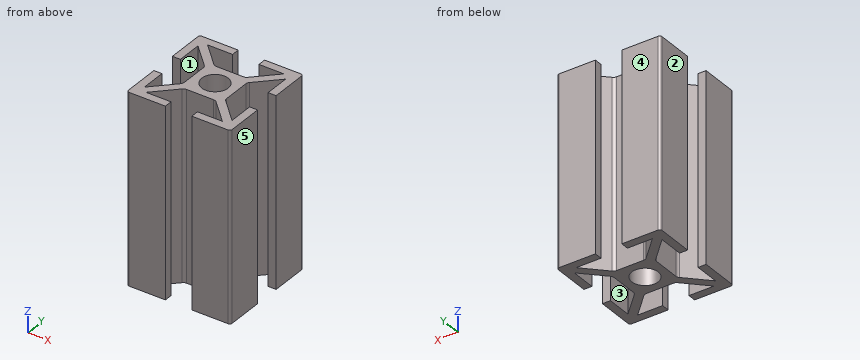
```python
from build123d import *

# Parameters (mm, degrees)
EXTRUSION1_DEPTH        = 40
ESQUISSE2_R             = 2.8
ENL_V_MAT_EXTRU_1_DEPTH = 41
CONG_1_R                = 0.5
CONG_2_R                = 1


with BuildPart() as part:
    # Esquisse1 → Extrusion1 (new body)
    with BuildSketch(Plane.XY):
        Polygon((-2.8, 11), (-2.8, 9.3), (-8.097918472, 9.3), (-3.297918472, 4.5), (3.297918472, 4.5), (8.097918472, 9.3), (2.8, 9.3), (2.8, 11), (11, 11), (11, 2.8), (9.3, 2.8), (9.3, 8.097918472), (4.5, 3.297918472), (4.5, -3.297918472), (9.3, -8.097918472), (9.3, -2.8), (11, -2.8), (11, -11), (2.8, -11), (2.8, -9.3), (8.097918472, -9.3), (3.297918472, -4.5), (-3.297918472, -4.5), (-8.097918472, -9.3), (-2.8, -9.3), (-2.8, -11), (-11, -11), (-11, -2.8), (-9.3, -2.8), (-9.3, -8.097918472), (-4.5, -3.297918472), (-4.5, 3.297918472), (-9.3, 8.097918472), (-9.3, 2.8), (-11, 2.8), (-11, 11), align=None)
    extrude(amount=EXTRUSION1_DEPTH)

    # Esquisse2 → Enlèv. mat.-Extru.1 (cut, through all)
    with BuildSketch(Plane(origin=(0, 0, 0), x_dir=(-1, 0, 0), z_dir=(0, 0, -1))):
        Circle(ESQUISSE2_R)
    extrude(amount=-ENL_V_MAT_EXTRU_1_DEPTH, mode=Mode.SUBTRACT)

    # Congé1
    cong_1_edges = [part.edges().sort_by_distance(p)[0] for p in [
        (-11, 11, 20),
        (11, 11, 20),
        (11, -11, 20),
        (-11, -11, 20),
    ]]
    fillet(cong_1_edges, radius=CONG_1_R)

    # Congé2
    cong_2_edges = [part.edges().sort_by_distance(p)[0] for p in [
        (-4.5, -3.297918472, 20),
        (-4.5, 3.297918472, 20),
        (-3.297918472, 4.5, 20),
        (3.297918472, 4.5, 20),
        (4.5, 3.297918472, 20),
        (4.5, -3.297918472, 20),
        (3.297918472, -4.5, 20),
        (-3.297918472, -4.5, 20),
    ]]
    fillet(cong_2_edges, radius=CONG_2_R)


solid = part.part
```
The model under review builds one solid part; all positions refer to its coordinate system, in mm. Face numbers are marked on the shaded views. A direction names the side the tool comes from. Round coordinates to 2 decimals unless told otherwise and drop trailing zeros. Loops run counter-clockwise (first coordinate to the right, second up) from the corner with the lowest first, then second, coordinate; pieces in that order, holes last. Notation, with made-up numbers: (76, -36.75) -> (110, -36.75) arc R12 ccw to (110, -32.75) -> close; hole circle Ø8 at (-0.75, -32.75). An arc over 180 degrees is marked (long way). Answer as a JSON object with one key per item and string values. Group by question number.
1) We need section C-C on x = -4. Write out the cut boundary in (y, z), then the cut area to 3 significant figures.
2) We need section D-D on y = -6.25. Write out the cut boundary in (x, z).
3) For line 1 (Y direction, x = 0, z = 21); line 2 (Y direction, x = 4.75, z = 22); line 3 (Y direction, x = -3.75, z = 33.5), list the stretches that pass through material, from the lowest coordinate up. Write a range as [from, to].
4) For the marked faces 1 and 2, list the 3-axis set-ups (+Z, -Z, +X, -X, +Y, -Y) from which the entire face can be reached by the end or side of a thin tool; tool diameter is ignored.
5) For pin 1 Ø3 at (x, z) = (1, 27.5) entering from -Y, flat-tipped, find the tip position at first contact; note if it passes through.
6) We need section A-A on y = 0. Write out the cut boundary in (x, z), then the cut area to 3 significant figures.
7) Mouldability with a two-part tool opening along X and no side actions: class the marked faces 3, 4 and 5 as released by +X, released by -X, zero draft, split by the parting line, or undercut.
Result set:
{
 "1": {"outline": "(-11, 0) -> (-9.3, 0) -> (-9.3, 40) -> (-11, 40) -> close; (-5.2, 0) -> (5.2, 0) -> (5.2, 40) -> (-5.2, 40) -> close; (9.3, 0) -> (11, 0) -> (11, 40) -> (9.3, 40) -> close", "area": "552 mm²"},
 "2": {"outline": "(-11, 0) -> (-9.3, 0) -> (-9.3, 40) -> (-11, 40) -> close; (-7.45, 0) -> (-5.05, 0) -> (-5.05, 40) -> (-7.45, 40) -> close; (5.05, 0) -> (7.45, 0) -> (7.45, 40) -> (5.05, 40) -> close; (9.3, 0) -> (11, 0) -> (11, 40) -> (9.3, 40) -> close"},
 "3": {"line 1": "[-4.5, -2.8], [2.8, 4.5]", "line 2": "[-11, -9.3], [-5.95, -3.55], [3.55, 5.95], [9.3, 11]", "line 3": "[-11, -9.3], [-4.95, 4.95], [9.3, 11]"},
 "4": {"face 1": "+Z, -Z", "face 2": "+Z, -Z, -X, +Y, -Y"},
 "5": {"pin 1": "y = -4.5"},
 "6": {"outline": "(-4.5, 0) -> (-2.8, 0) -> (-2.8, 40) -> (-4.5, 40) -> close; (2.8, 0) -> (4.5, 0) -> (4.5, 40) -> (2.8, 40) -> close", "area": "136 mm²"},
 "7": {"face 3": "undercut", "face 4": "zero draft", "face 5": "released by +X"}
}
